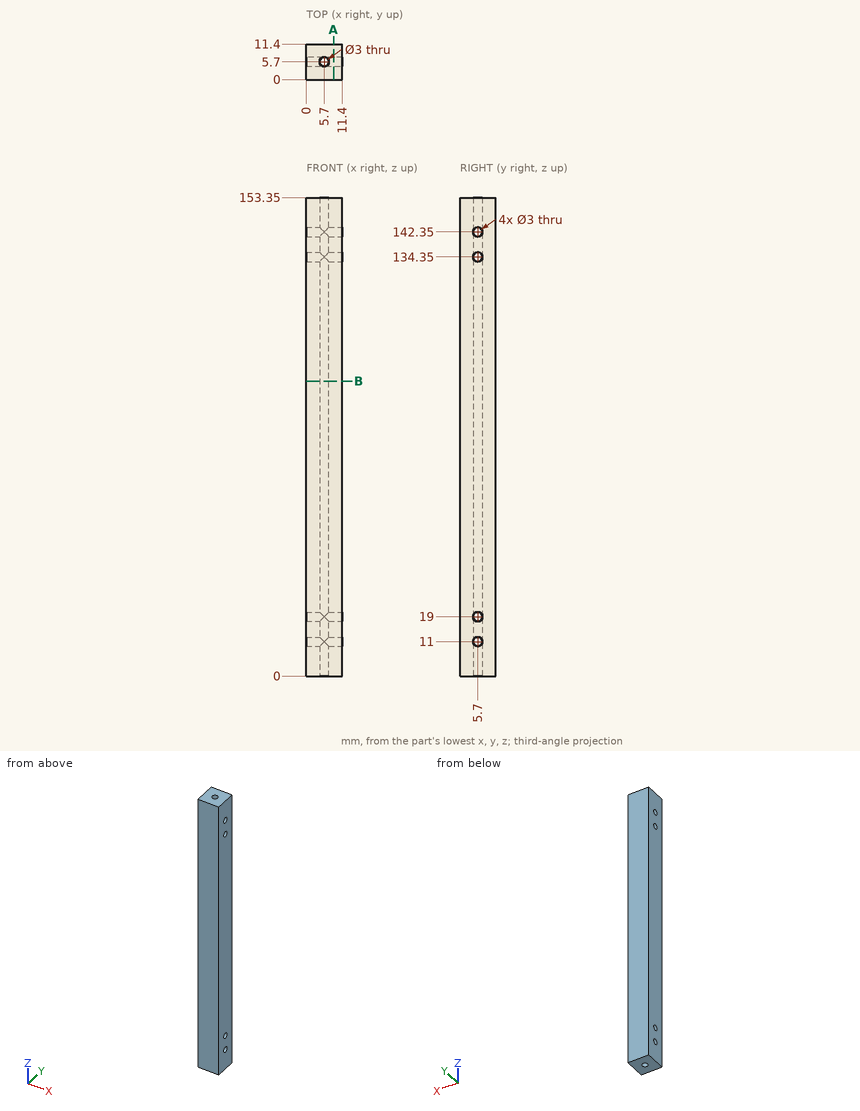
Input: dimensioned drawing with shaded views. Units: mm. Origin: part minimum x, y, z. Give positions to 0.01 mm unless a question says otherwise; leave off trailing zeros. Loops run counter-clockwise (first coordinate to the right, second up) from the corner with the lowest first, then second, coordinate; pieces in that order, holes last. Notation, with made-up numbers: (-11.75, -5) -> (47.25, -5) arc R27 cw to (47.25, 22) -> close; hole circle Ø10 at (71, 6.25). An arc over 180 degrees is marked (long way). Use a Markdown table: item, result.
Q1. Section query B-B, the plane z = 94.5. Return the cut outline in (x, y), plus the area to 3 significant figures.
Entries:
| item | result |
|---|---|
| outline | (0, 0) -> (11.4, 0) -> (11.4, 11.4) -> (0, 11.4) -> close; hole circle Ø3 at (5.7, 5.7) |
| area | 123 mm² |
Q2. Section query A-A, the plane x = 8.75. Return the cut outline in (y, z), plus the area to 3 significant figures.
Entries:
| item | result |
|---|---|
| outline | (0, 0) -> (11.4, 0) -> (11.4, 153.35) -> (0, 153.35) -> close; hole circle Ø3 at (5.7, 11); hole circle Ø3 at (5.7, 19); hole circle Ø3 at (5.7, 134.35); hole circle Ø3 at (5.7, 142.35) |
| area | 1,720 mm² |
Q3. Ray query, probe 1 along Z at (x, y) = (8.85, 5.7); probe 2 along Y at (x, z) = (5.7, 137.75); probe 3 along Y at (x, z) = (6.25, 51). Return the intervals inside material, ascending. Write a range as from..to.
Entries:
| item | result |
|---|---|
| probe 1 | z = 0..9.5, 12.5..17.5, 20.5..132.85, 135.85..140.85, 143.85..153.35 |
| probe 2 | y = 0..4.2, 7.2..11.4 |
| probe 3 | y = 0..4.3, 7.1..11.4 |
